```python
from build123d import *

# Parameters (mm, degrees)
CROQUIS1_W              = 203.2
CROQUIS1_H              = 139.7
SALIENTE_EXTRUIR1_DEPTH = 50.8
CROQUIS2_W              = 165.1
CROQUIS2_H              = 38.1
CORTAR_EXTRUIR1_DEPTH   = 181.05357536
CROQUIS3_R              = 11.1125
CORTAR_EXTRUIR2_DEPTH   = 181.05357536
REDONDEO1_R             = 12.7
REDONDEO2_R             = 12.7
REDONDEO3_R             = 2.4


with BuildPart() as part:
    # Croquis1 → Saliente-Extruir1 (new body)
    with BuildSketch(Plane.XY):
        Rectangle(CROQUIS1_W, CROQUIS1_H)
    extrude(amount=SALIENTE_EXTRUIR1_DEPTH)

    # Croquis2 → Cortar-Extruir1 (cut, through all)
    with BuildSketch(Plane.XZ.offset(69.85)):
        with Locations((19.05, 31.75)):
            Rectangle(CROQUIS2_W, CROQUIS2_H)
    extrude(amount=-CORTAR_EXTRUIR1_DEPTH, mode=Mode.SUBTRACT)

    # Croquis3 → Cortar-Extruir2 (cut, through all)
    with BuildSketch(Plane.XZ.offset(69.85)):
        with Locations(Location((-82.55, 25.4, 0), (0, 0, 270))):
            Circle(CROQUIS3_R)
    extrude(amount=-CORTAR_EXTRUIR2_DEPTH, mode=Mode.SUBTRACT)

    # Redondeo1
    redondeo1_edges = [part.edges().sort_by_distance(p)[0] for p in [
        (-101.6, 0, 50.8),
        (-63.5, 0, 12.7),
        (-63.5, 0, 50.8),
    ]]
    fillet(redondeo1_edges, radius=REDONDEO1_R)

    # Redondeo2
    redondeo2_edges = [part.edges().sort_by_distance(p)[0] for p in [
        (101.6, -69.85, 6.35),
        (101.6, 69.85, 6.35),
    ]]
    fillet(redondeo2_edges, radius=REDONDEO2_R)

    # Redondeo3
    redondeo3_edges = [part.edges().sort_by_distance(p)[0] for p in [
        (-82.55, 69.85, 50.8),
        (-82.55, -69.85, 50.8),
        (19.05, -69.85, 12.7),
        (-63.5, -69.85, 31.75),
        (-101.6, -69.85, 19.05),
        (-67.219743879, -69.85, 47.080256121),
        (-97.880256121, -69.85, 47.080256121),
        (-101.6, 69.85, 19.05),
        (-63.5, 69.85, 31.75),
        (19.05, 69.85, 12.7),
        (-67.219743879, 69.85, 47.080256121),
        (-97.880256121, 69.85, 47.080256121),
        (-59.780256121, -69.85, 16.419743879),
        (-59.780256121, 69.85, 16.419743879),
        (-6.35, -69.85, 0),
        (-6.35, 69.85, 0),
        (101.6, 0, 0),
        (-101.6, 0, 0),
        (97.880256121, -66.130256121, 0),
        (97.880256121, 66.130256121, 0),
        (101.6, 0, 12.7),
        (97.880256121, -66.130256121, 12.7),
        (97.880256121, 66.130256121, 12.7),
    ]]
    fillet(redondeo3_edges, radius=REDONDEO3_R)


solid = part.part
```
Input: part model. Units: mm. Frame: model coordinates. A direction names the side the tool comes from. Round coordinates to 2 decimals unless told otherwise and drop trailing zeros. Order: outer loops, then holes, each group sorted by start corner. A loop starts at its lowest first (then second) coordinate and runs counter-clockwise, first axis right, second up. Notation, with made-up numbers: (19.25, 24.5) - (30.25, 24.5) arc R3 ccw to (30.25, 29.5) - close; hole circle Ø5 at (-33, 10.5). An arc over 180 degrees is marked (long way). Answer in a Markdown table with one row per item.
Item 1: Reachability of faces 1 (the flat face through (23, -1, 12.7)), 2 (the cylindrical face through (97.78, 66.23, 6.41)) from +Z, -Z, +X, -X, +Y, -Y: full face, straight path, thin tool, end or side. Return the list, or none.
Model answer:
| item | result |
|---|---|
| face 1 | +Z, +X, +Y, -Y |
| face 2 | +Z, -Z, +X, +Y |
Item 2: Pin query (flat end, axial travel): pin 1 (10 mm diameter, centred on x = 45.5, y = 6.5, fed in from +Z); pin 2 (3 mm diameter, centred on y = 55.5, z = 18, fed in from +X); pin 3 (5 mm diameter, centred on x = -28, z = 17, fed in from +Y); pin 4 (4 mm diameter, centred on y = -6, z = 31, fed in from +X). Return the tip coordinate at first contact, or that it passes through.
Model answer:
| item | result |
|---|---|
| pin 1 | stops at z = 12.7 |
| pin 2 | stops at x = -59.86 |
| pin 3 | passes through |
| pin 4 | stops at x = -63.5 |
Item 3: Section query C-C (x = 11.5). Return the cut outline in (y, z).
Model answer:
| item | result |
|---|---|
| outline | (-69.85, 2.4) arc R2.4 ccw to (-67.45, 0) - (67.45, 0) arc R2.4 ccw to (69.85, 2.4) - (69.85, 10.3) arc R2.4 ccw to (67.45, 12.7) - (-67.45, 12.7) arc R2.4 ccw to (-69.85, 10.3) - close |
Item 4: Section query A-A (x = -82.55). Return the cut outline in (y, z), then the cut area to 3 significant figures.
Model answer:
| item | result |
|---|---|
| outline | (-69.85, 2.4) arc R2.4 ccw to (-67.45, 0) - (67.45, 0) arc R2.4 ccw to (69.85, 2.4) - (69.85, 14.29) - (-69.85, 14.29) - close; (-69.85, 36.51) - (69.85, 36.51) - (69.85, 48.4) arc R2.4 ccw to (67.45, 50.8) - (-67.45, 50.8) arc R2.4 ccw to (-69.85, 48.4) - close |
| area | 3,990 mm² |
Item 5: Line query: line 1 (X direction, y = 33, z = 25); line 2 (Z direction, x = 16, y = -56); line 3 (X direction, y = -44, z = 37.5). Output: solid intervals per line, ascending.
Model answer:
| item | result |
|---|---|
| line 1 | x = -101.6 to -93.66, -71.44 to -63.49 |
| line 2 | z = 0 to 12.7 |
| line 3 | x = -101.6 to -63.5 |
Item 6: Mould query, pull axis X, two halves, no side actions, for faces 3 (the cylindrical face through (-71.532, -0.978, 26.847)), 4 (the cylindrical face through (-97.98, 0.94, 46.98)), 5 (the cylindrical face through (-67.32, 0.94, 47.18)). Classes: released by +X, released by -X, zero draft, split by the parting line, or undercut.
Model answer:
| item | result |
|---|---|
| face 3 | undercut |
| face 4 | released by -X |
| face 5 | released by +X |
Item 7: Section query D-D (z = 31). Return the cut outline in (x, y), then the cut area to 3 significant figures.
Model answer:
| item | result |
|---|---|
| outline | (-101.6, -67.45) arc R2.4 ccw to (-99.2, -69.85) - (-92.15, -69.85) - (-92.15, 69.85) - (-99.2, 69.85) arc R2.4 ccw to (-101.6, 67.45) - close; (-72.95, -69.85) - (-65.9, -69.85) arc R2.4 ccw to (-63.5, -67.45) - (-63.5, 67.45) arc R2.4 ccw to (-65.9, 69.85) - (-72.95, 69.85) - close |
| area | 2,640 mm² |
